Autodesk Inventor part; units mm, degrees
ref_plane "YZ Plane" through (0, 0, 0) normal (1, 0, 0) x (0, 1, 0)
ref_plane "XZ Plane" through (0, 0, 0) normal (0, 1, 0) x (-1, 0, 0)
ref_plane "XY Plane" through (0, 0, 0) normal (0, 0, 1) x (1, 0, 0)
sketch "Sketch1" plane through (0, 0, 0) normal (0, 0, 1) x (1, 0, 0)
  circle A0 centre (10, 20.7) radius 1.6
  line L0 (0, 0) -> (20.0001, 0)
  line L1 (0, 0) -> (0, 7)
  line L2 (20.0001, 0) -> (20.0001, 6.9998)
  line L3 (0, 7) -> (5.4723, 22.0351)
  line L4 (0, 7) -> (16, 7) construction
  line L5 (20.0001, 6.9998) -> (14.5277, 22.0349)
  line L6 (20.0001, 6.9998) -> (36.0001, 6.9998) construction
  arc A1 (14.5277, 22.0349) -> (5.4723, 22.0351) centre (10, 20.3869) ccw
  dimension "d17" = 7
  dimension "d18" = 6.9998
  dimension "d19" = 20.7
  dimension "d23" = 90
  dimension "d24" = 90
  dimension "d25" = 10
  dimension "d26" = 16
  dimension "d27" = 70
  dimension "d28" = 16
  dimension "d29" = 110
  dimension "d30" = 10
sketch "Sketch3" plane through (0, 0, 0) normal (0, 0, 1) x (1, 0, 0)
  point P0 (0, 0)
extrude "Extrusion1" add sketch "Sketch1" along normal blind 4.2
sketch "Sketch4" plane through (0, 0, 4.2) normal (0, 0, 1) x (1, 0, 0)
  line L0 (0, 7) -> (0, 0)
  line L1 (20.0001, 0) -> (20.0001, 6.9998)
  line L2 (0, 0) -> (20.0001, 0)
  line L3 (20.0001, 0) -> (20.0001, 6.9998)
  line L4 (3.884, 22.9404) -> (-0.0481, 7.0119)
  line L5 (20.0001, 6.9998) -> (0, 6.9998)
  line L6 (0, 7) -> (0, 0)
extrude "Extrusion2" add sketch "Sketch4" along normal blind 4.2
sketch "Sketch5" plane through (0, 0, 0) normal (0, -1, 0) x (1, 0, 0)
  circle A0 centre (5, 3.6) radius 0.5
  circle A1 centre (15, 3.6) radius 0.5
  line L0 (0, 0) -> (20.0001, 0)
  line L1 (0, 8.4) -> (20.0001, 8.4)
  dimension "d13" = 1
  dimension "d14" = 1
  dimension "d33" = 4.8
  dimension "d34" = 4.8
extrude "Extrusion3" cut sketch "Sketch5" against normal blind 5.5
properties part number "upper_deck_shaft_mount_v3"
Part model, mm, in its own coordinate system. A direction names the side the tool comes from. Round coordinates to 2 decimals unless told otherwise and drop trailing zeros. Write each loop counter-clockwise with the first axis right and the second up, starting at its lowest first coordinate (ties: lowest second). Pieces come first, ordered by that corner, then holes. Notation, with made-up numbers: (29, 81.25) -> (61, 81.25) arc R13 cw to (61, 102.25) -> close; hole circle Ø5 at (26.25, 16). An arc over 180 degrees is marked (long way). Return JSON: item names as keys, results as strings. Group by question number.
Q1. Saw through at D-D on z = 2.25. Write the cut outline in (x, y).
Q2. Saw through at C-C on y = 20.7. Write the cut outline in (x, z).
Q3. Pin check, flat tips, straight feed: pin 1 (6 mm diameter, centred on x = 7.5, y = 11.5, fed in from +Z); pin 2 (2 mm diameter, centred on x = 13, z = 6.5, fed in from +Y). Stop position of each tip, or through.
Q4. Saw through at B-B on x = 10. Write the cut outline in (y, z).
Q5. Mould opens along Y. For faces 1 (the cylindrical face through (8.73, 21.67, 2.07)), 2 (the cylindrical face through (9.918, 25.204, 2.071)), 3 (the flat face through (10, 14, 4.2)), 4 (the flat face through (5, 5.5, 3.6)) say: pulls with the +Y half, pulls with the -Y half, needs draft (parallel to the pull), parting line crosses it, or undercut.
Q6. Which spindle directions (+Z, -Z, +X, -X, +Y, -Y) get a long thin tool onto all of the face, cutting with end or side? Do faces 5 (the flat face through (15, 5.5, 3.6)), 6 (the flat face through (2.698, 14.412, 2.071)). Say none if no direction does.
Q7. Probe L1, parallel to Z at x = 15, y = 3.5; L2, parallel to Y at x = 4, z = 6.75; L3, parallel to Z at x = 9.5, y = 18.75. List the from-to ranges inside material, lowest first. Write a range as [from, to].
Q8. Saw through at A-A on z = 3.6. Write the cut outline in (x, y).
Answer:
{
 "1": {"outline": "(0, 0) -> (20, 0) -> (20, 7) -> (14.53, 22.03) arc R4.82 ccw to (5.47, 22.04) -> (0, 7) -> close; hole circle Ø3.2 at (10, 20.7)"},
 "2": {"outline": "(4.99, 0) -> (8.4, 0) -> (8.4, 4.2) -> (4.99, 4.2) -> close; (11.6, 0) -> (15.01, 0) -> (15.01, 4.2) -> (11.6, 4.2) -> close"},
 "3": {"pin 1": "z = 4.2", "pin 2": "y = 7"},
 "4": {"outline": "(0, 0) -> (19.1, 0) -> (19.1, 4.2) -> (7, 4.2) -> (7, 8.4) -> (0, 8.4) -> close; (22.3, 0) -> (25.21, 0) -> (25.21, 4.2) -> (22.3, 4.2) -> close"},
 "5": {"face 1": "undercut", "face 2": "pulls with the +Y half", "face 3": "needs draft", "face 4": "pulls with the -Y half"},
 "6": {"face 5": "-Y", "face 6": "+Z, -Z, -X, +Y"},
 "7": {"L1": "[0, 3.1], [4.1, 8.4]", "L2": "[0, 7]", "L3": "[0, 4.2]"},
 "8": {"outline": "(0, 0) -> (4.5, 0) -> (4.5, 5.5) -> (5.5, 5.5) -> (5.5, 0) -> (14.5, 0) -> (14.5, 5.5) -> (15.5, 5.5) -> (15.5, 0) -> (20, 0) -> (20, 7) -> (14.53, 22.03) arc R4.82 ccw to (5.47, 22.04) -> (0, 7) -> close; hole circle Ø3.2 at (10, 20.7)"}
}
